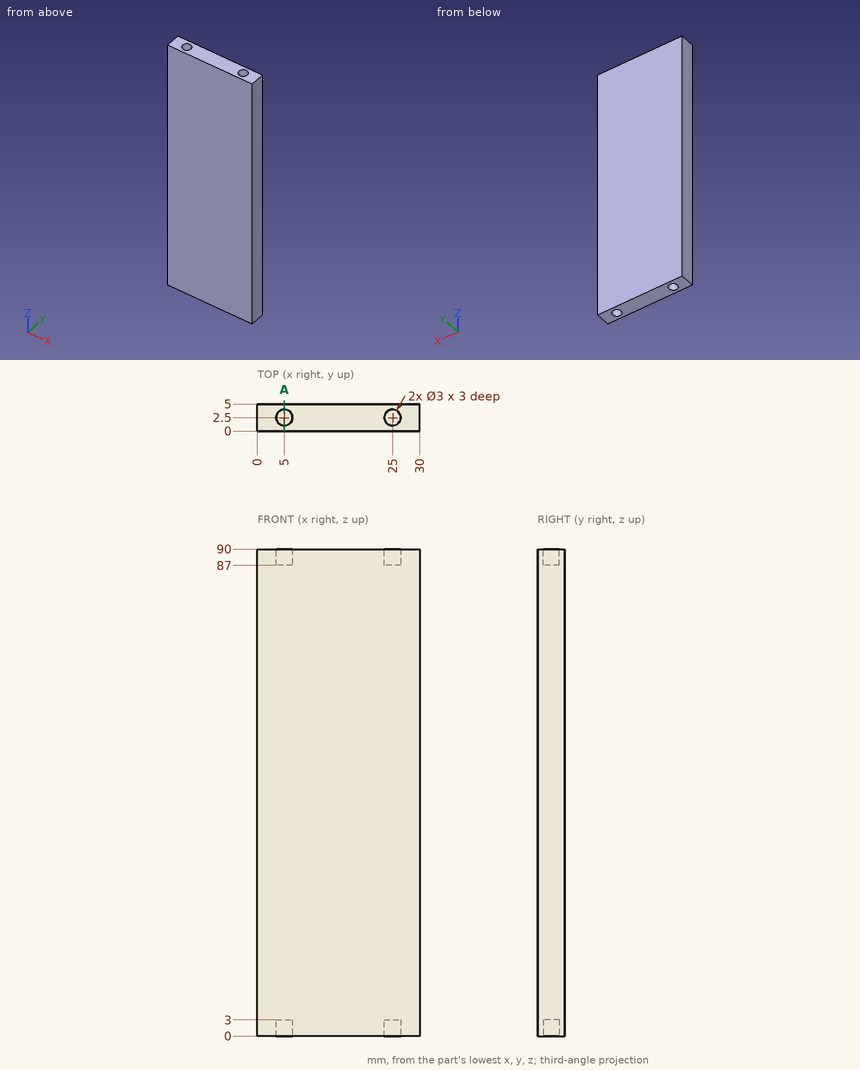
For this review, use the dimensioned drawing (mm, ordinates from the lowest corner) and the shaded views. Give positions to 0.01 mm unless a question says otherwise; leave off trailing zeros. Order: outer loops, then holes, each group sorted by start corner. A loop starts at its lowest first (then second) coordinate and runs counter-clockwise, first axis right, second up. Notation, with made-up numbers: M 82,36.25 L 108,36.25 A24 ccw 108,64.25 Z; hole C -8.75,-12.75 d11. An arc over 180 degrees is marked long. One line per question, with ' | ' between items. Start each with the question number.
1) Consider section A-A, the plane x = 5. Give the boundary of the cut face in (y, z).
2) Clearance check with flat-ended pins moving along their axes: P1, Ø0.9, axis at x = 5, y = 2.5, coming from the +Z side; P2, Ø1.5, axis at x = 5.5, y = 2, coming from the -Z side. State where each tip first meets the part, or that it passes through.
3) Wall thickness on L1, parallel to Y at x = 25, z = 89.45; L2, parallel to Z at x = 25, y = 2.35: over which ranges is each line inside the solid? List them lowest first. Write a range as from..to.
Found:
1) outline: M 0,0 L 1,0 L 1,3 L 4,3 L 4,0 L 5,0 L 5,90 L 4,90 L 4,87 L 1,87 L 1,90 L 0,90 Z
2) P1: stops at z = 87 | P2: stops at z = 3
3) L1: y = 0..1, 4..5 | L2: z = 3..87
